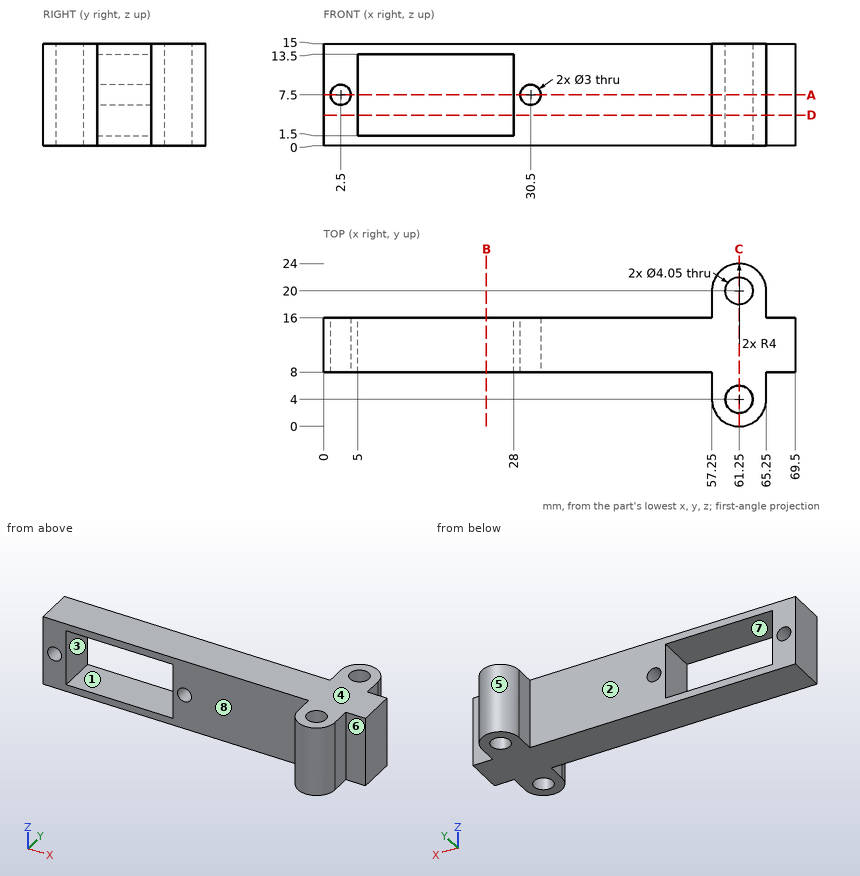
Drawing for the job (mm, zero at the part's lowest x, y, z). A direction names the side the tool comes from. Coordinates: 2 decimals unless noted, no trailing zeros. Order: outer loops, then holes, each group sorted by start corner. A loop starts at its lowest first (then second) coordinate and runs counter-clockwise, first axis right, second up. Notation, with made-up numbers: (25, 75.5) -> (40, 75.5) arc R13 cw to (40, 88.5) -> close; hole circle Ø2 at (65, -16.75). An arc over 180 degrees is marked (long way). Answer in a Markdown table with one row per item.
1) Band-saw the part on A-A (z = 7.5). List the corners of the cut face in (x, y) (3 decimals).
Check values:
| item | result |
|---|---|
| outline | (0, 8) -> (1, 8) -> (1, 16) -> (0, 16) -> close; (4, 8) -> (5, 8) -> (5, 16) -> (4, 16) -> close; (28, 8) -> (29, 8) -> (29, 16) -> (28, 16) -> close; (32, 8) -> (57.25, 8) -> (57.25, 4) arc R4 ccw to (65.25, 4) -> (65.25, 8) -> (69.5, 8) -> (69.5, 16) -> (65.25, 16) -> (65.25, 20) arc R4 ccw to (57.25, 20) -> (57.25, 16) -> (32, 16) -> close; hole circle Ø4.05 at (61.25, 4); hole circle Ø4.05 at (61.25, 20) |
2) Drill centre lines: line 1 (Y direction, x = 61.25, z = 9) (3 decimals); line 2 (X direction, y = 10.25, z = 7.5); line 3 (X direction, y = 13.5, z = 7). Where is each one in solid material? Low to high.
Check values:
| item | result |
|---|---|
| line 1 | 0 to 1.975, 6.025 to 17.975, 22.025 to 24 |
| line 2 | 0 to 1, 4 to 5, 28 to 29, 32 to 69.5 |
| line 3 | 0 to 1.09, 3.91 to 5, 28 to 29.09, 31.91 to 69.5 |
3) Band-saw the part on D-D (z = 4.5). List the corners of the cut face in (x, y) (3 decimals), and give its area (4 significant figures).
Check values:
| item | result |
|---|---|
| outline | (0, 8) -> (5, 8) -> (5, 16) -> (0, 16) -> close; (28, 8) -> (57.25, 8) -> (57.25, 4) arc R4 ccw to (65.25, 4) -> (65.25, 8) -> (69.5, 8) -> (69.5, 16) -> (65.25, 16) -> (65.25, 20) arc R4 ccw to (57.25, 20) -> (57.25, 16) -> (28, 16) -> close; hole circle Ø4.05 at (61.25, 4); hole circle Ø4.05 at (61.25, 20) |
| area | 460.5 mm2 |
4) Mould opens along Z. For the marked faces 1, 2, 3 and 4 say: pulls with the +Z half, pulls with the -Z half, needs draft (parallel to the pull), parting line crosses it, or undercut.
Check values:
| item | result |
|---|---|
| face 1 | undercut |
| face 2 | needs draft |
| face 3 | undercut |
| face 4 | pulls with the +Z half |
5) Band-saw the part on C-C (x = 61.25). List the corners of the cut face in (y, z) (3 decimals).
Check values:
| item | result |
|---|---|
| outline | (0, 0) -> (1.975, 0) -> (1.975, 15) -> (0, 15) -> close; (6.025, 0) -> (17.975, 0) -> (17.975, 15) -> (6.025, 15) -> close; (22.025, 0) -> (24, 0) -> (24, 15) -> (22.025, 15) -> close |
6) Flat gauge pins, fed straight in: P1, Ø4, axis at y = 5.5, z = 9, coming from the +X side; P2, Ø2, axis at y = 18, z = 10, coming from the -X side; P3, Ø3.5, axis at x = 2.5, z = 7.5, coming from the +Y side. Where does each tip first touch, or does it go through?
Check values:
| item | result |
|---|---|
| P1 | x = 65.25 |
| P2 | x = 57.25 |
| P3 | y = 16 |
7) Which spindle directions (+Z, -Z, +X, -X, +Y, -Y) get a long thin tool onto all of the face, cutting with end or side? Do the marked faces 5, 6, 7 and 8. Say none if no direction does.
Check values:
| item | result |
|---|---|
| face 5 | +Z, -Z, +Y |
| face 6 | +Z, -Z, +X, -Y |
| face 7 | +Y, -Y |
| face 8 | +Z, -Z, -X, -Y |
8) Band-saw the part on B-B (x = 24). List the corners of the cut face in (y, z), and give its area (3 significant figures).
Check values:
| item | result |
|---|---|
| outline | (8, 0) -> (16, 0) -> (16, 1.5) -> (8, 1.5) -> close; (8, 13.5) -> (16, 13.5) -> (16, 15) -> (8, 15) -> close |
| area | 24.0 mm2 |
